Could you check a few things on this model? Use its own coordinates, in mm. A direction names the side the tool comes from. Coordinates: 2 decimals unless noted, no trailing zeros. Order: outer loops, then holes, each group sorted by start corner. A loop starts at its lowest first (then second) coordinate and runs counter-clockwise, first axis right, second up. Notation, with made-up numbers: (-26, 17.25) -> (-9, 17.25) arc R15 cw to (-9, 44.25) -> close; hole circle Ø6 at (5.5, 7). An arc over 180 degrees is marked (long way). Use a Markdown table: item, result. Add a question column.
1) Thinking about a two-plate mould opening in Y: for faces 4 (the conical face through (-17.716, 17.504, 7.141)), 5 (the cylindrical face through (-11.43, 20.6, 13.51)), 6 (the flat face through (0, -15, 14)), 7 (the conical face through (14.91, -30.71, 13.86)), which applies, +Y half, -Y half, draft (parallel to the pull), parting line (faces both ways), or undercut?
2) If we section it at A-A (x = 0): Write out the boundary of the cut face in (y, z), plus the area to 3 significant figures.
3) If I drill on L1, parallel to X at y = -11.5, z = 3.75; L2, parallel to Y at x = -9.5, z = 5.5; L3, parallel to X at y = 8.5, z = 11.5, over which ranges is the centre line in solid material (lowest first)? Write a range as [from, to].
4) If we section it at B-B (z = 4.5): Write out the boundary of the cut face in (x, y).
5) If we section it at C-C (z = 8.5): Give the number of separate pieces and of enclosed holes in the cut face, plus the area to 3 significant figures.
6) Will these pins go through, and if not, where does the flat tip stop? pin 1 Ø4 at (x, z) = (5, 8.5) entering from +Y; pin 2 Ø5 at (x, z) = (-27, 9) entering from -Y; pin 3 Ø1.6 at (x, y) = (-17.68, -17.68) entering from +Z.
7) Which directions (+Z, -Z, +X, -X, +Y, -Y) give clear straight access to the entire face, cutting with the end or side of a thin tool? Please do faces 1 (the flat face through (-27.921, 16.977, 13.014)), 2 (the flat face through (25.4, 15.5, 10)), 3 (the cylindrical face through (-17.54, -16.66, 10.78)).
```python
from build123d import *

# Parameters (mm, degrees)
SKETCH1_R               = 29.5
BOSS_EXTRUDE1_DEPTH     = 10
SKETCH2_R               = 34.5
BOSS_EXTRUDE2_DEPTH     = 4
SKETCH3_R               = 12.5
CUT_EXTRUDE1_DEPTH      = 15
M4_TAPPED_HOLE1_D       = 3.3
M2_5_TAPPED_HOLE1_D     = 2.05
M2_5_TAPPED_HOLE1_DEPTH = 6.35
M2_5_TAPPED_HOLE1_TIP   = 0.615882135
CHAMFER1_SIZE           = 0.5
CUT_EXTRUDE2_DEPTH      = 2
CUT_EXTRUDE4_DEPTH      = 1


with BuildPart() as part:
    # Sketch1 → Boss-Extrude1 (new body)
    with BuildSketch(Plane.XY):
        Circle(SKETCH1_R)
    extrude(amount=BOSS_EXTRUDE1_DEPTH)

    # Sketch2 → Boss-Extrude2 (add)
    with BuildSketch(Plane.XY.offset(10)):
        Circle(SKETCH2_R)
    extrude(amount=BOSS_EXTRUDE2_DEPTH)

    # Sketch3 → Cut-Extrude1 (cut, through all)
    with BuildSketch(Plane.XY.offset(14)):
        Circle(SKETCH3_R)
    extrude(amount=-CUT_EXTRUDE1_DEPTH, mode=Mode.SUBTRACT)

    # M4 Tapped Hole1 (through all)
    with Locations(Plane.XY.offset(14)):
        with Locations((-10.606601718, 10.606601718), (10.606601718, 10.606601718), (10.606601718, -10.606601718), (-10.606601718, -10.606601718)):
            Hole(M4_TAPPED_HOLE1_D / 2)

    # M2.5 Tapped Hole1
    with Locations(Plane.XY.offset(14)):
        with Locations((-17.67766953, -17.67766953), (-25, 0), (-17.67766953, 17.67766953)):
            Hole(M2_5_TAPPED_HOLE1_D / 2, depth=M2_5_TAPPED_HOLE1_DEPTH)
            with Locations((0, 0, -(M2_5_TAPPED_HOLE1_DEPTH + M2_5_TAPPED_HOLE1_TIP / 2))):  # 118° drill point
                Cone(0, M2_5_TAPPED_HOLE1_D / 2, M2_5_TAPPED_HOLE1_TIP, mode=Mode.SUBTRACT)

    # Chamfer1
    chamfer1_edges = [part.edges().sort_by_distance(p)[0] for p in [
        (-34.5, 0, 14),
    ]]
    chamfer(chamfer1_edges, length=CHAMFER1_SIZE)

    # Sketch9 → Cut-Extrude2 (cut)
    with BuildSketch(Plane.XY.offset(14)):
        with BuildLine():
            Line((-33.450745653, 8.44379152), (-30.091742903, 7.052447025))
            ThreePointArc((-30.091742903, 7.052447025), (-29.326376039, 7.052447025), (-28.785179939, 7.593643125))
            Line((-28.785179939, 7.593643125), (-25.72371248, 14.984679385))
            ThreePointArc((-25.72371248, 14.984679385), (-25.72371248, 15.75004625), (-26.26490858, 16.29124235))
            Line((-26.26490858, 16.29124235), (-29.62391133, 17.682586845))
            ThreePointArc((-29.62391133, 17.682586845), (-31.873843872, 13.202578417), (-33.450745653, 8.44379152))
        make_face()
    extrude(amount=-CUT_EXTRUDE2_DEPTH, mode=Mode.SUBTRACT)

    # Sketch11 → Cut-Extrude4 (cut)
    with BuildSketch(Plane.XY.offset(14)):
        with BuildLine():
            Line((-12, 32.345787979), (-12, 22))
            ThreePointArc((-12, 22), (-11.414213562, 20.585786438), (-10, 20))
            Line((-10, 20), (10, 20))
            ThreePointArc((10, 20), (11.414213562, 20.585786438), (12, 22))
            Line((12, 22), (12, 32.345787979))
            ThreePointArc((12, 32.345787979), (0, 34.5), (-12, 32.345787979))
        make_face()
    extrude(amount=-CUT_EXTRUDE4_DEPTH, mode=Mode.SUBTRACT)


solid = part.part
```
Answer sheet:
| question | item | result |
|---|---|---|
| 1 | face 4 | undercut |
| 1 | face 5 | +Y half |
| 1 | face 6 | draft |
| 1 | face 7 | parting line |
| 2 | outline | (-34.5, 10) -> (-29.5, 10) -> (-29.5, 0) -> (-12.5, 0) -> (-12.5, 14) -> (-34, 14) -> (-34.5, 13.5) -> close; (12.5, 0) -> (29.5, 0) -> (29.5, 10) -> (34.5, 10) -> (34.5, 13) -> (20, 13) -> (20, 14) -> (12.5, 14) -> close |
| 2 | area | 501 mm2 |
| 3 | L1 | [-27.17, -11.99], [-9.22, -4.9], [4.9, 9.22], [11.99, 27.17] |
| 3 | L2 | [-27.93, -11.83], [-9.38, -8.12], [8.12, 9.38], [11.83, 27.93] |
| 3 | L3 | [-33.44, -9.17], [9.17, 33.44] |
| 4 | outline | circle Ø59 at (0, 0); hole circle Ø25 at (0, 0); hole circle Ø3.3 at (-10.61, -10.61); hole circle Ø3.3 at (-10.61, 10.61); hole circle Ø3.3 at (10.61, -10.61); hole circle Ø3.3 at (10.61, 10.61) |
| 5 | separate pieces | 1 |
| 5 | enclosed holes | 8 |
| 5 | area | 2,200 mm2 |
| 6 | pin 1 | y = 34.3 |
| 6 | pin 2 | y = -24.08 |
| 6 | pin 3 | z = 7.52 |
| 7 | face 1 | +Z, -X |
| 7 | face 2 | -Z |
| 7 | face 3 | +Z |
